```python
from build123d import *

# Parameters (mm, degrees)
BOSS_EXTRUDE1_DEPTH                           = 50.8
CSK_FOR_8_FLAT_HEAD_MACHINE_SCREW1_AT_2_COUNT = 2
CSK_FOR_8_FLAT_HEAD_MACHINE_SCREW1_AT_2_PITCH = 31.75


with BuildPart() as part:
    # Sketch1 → Boss-Extrude1 (new body)
    with BuildSketch(Plane.XY):
        Polygon((0, 0), (0, 38.1), (3.175, 38.1), (3.175, 3.175), (92.075, 3.175), (92.075, 25.4), (95.25, 25.4), (95.25, 0), align=None)
    extrude(amount=BOSS_EXTRUDE1_DEPTH)

    # Sketch3 → CSK for #8 Flat Head Machine Screw1 (revolve, cut)
    with BuildSketch(Plane(origin=(3.175, 31.75, 41.275), x_dir=(0, 0, -1), z_dir=(0, 1, 0))):
        Polygon((0, 0), (0, 3.175), (2.2479, 3.175), (2.2479, 2.26450021), (4.2164, 0), align=None)
    csk_for_8_flat_head_machine_screw1 = revolve(axis=Axis((9.525, 31.75, 41.275), (-1, 0, 0)), mode=Mode.SUBTRACT)

    # CSK for #8 Flat Head Machine Screw1 at 2: CSK for #8 Flat Head Machine Screw1 ×2
    with Locations(*[(0, 0, -i * CSK_FOR_8_FLAT_HEAD_MACHINE_SCREW1_AT_2_PITCH) for i in range(1, CSK_FOR_8_FLAT_HEAD_MACHINE_SCREW1_AT_2_COUNT)]):
        add(csk_for_8_flat_head_machine_screw1, mode=Mode.SUBTRACT)


solid = part.part
```
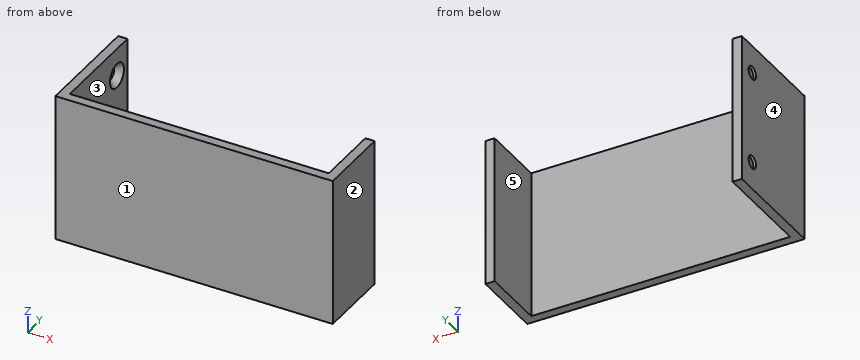
Source: CAD feature listing. Evaluate the final solid. Frame: model axes, mm. Face numbers are marked on the shaded views. A direction names the side the tool comes from. Give positions to 0.01 mm unless a question says otherwise; leave off trailing zeros. Loops run counter-clockwise (first coordinate to the right, second up) from the corner with the lowest first, then second, coordinate; pieces in that order, holes last. Notation, with made-up numbers: (19.5, -12.5) - (56.5, -12.5) arc R17 ccw to (56.5, 17.5) - close; hole circle Ø2 at (24.5, 21). An arc over 180 degrees is marked (long way). Use CSV: the item, a comma, the result in double quotes. Start each with the question number.
1. Section A-A (y = 31.75). Output: boundary loops of the cut face in (x, z) (1 decimal), then the cut area to 3 significant figures.
2. Section B-B (z = 35.5). Output: boundary loops of the cut face in (x, y) (3 decimals), then the cut area to 3 significant figures.
3. Draft query along X for the marked faces 1, 2 and 3. Return one class per face: +X half, -X half, draft (parallel to the pull), parting line (faces both ways), or undercut.
4. Ray query, L1, parallel to Z at x = 0.5, y = 31.75; L2, parallel to X at y = 11, z = 12.5 (3 decimals); L3, parallel to X at y = 35.5, z = 5 (3 decimals). Return the intervals inside material, ascending.
5. Section C-C (y = 4.5). Output: boundary loops of the cut face in (x, z) (3 decimals).
6. Reachability of the marked faces 4 and 5 from +Z, -Z, +X, -X, +Y, -Y: full face, straight path, thin tool, end or side. Return the list, or none.
7. Pin query (flat end, axial travel): pin 1 (2.5 mm diameter, centred on x = 94, z = 29, fed in from +Y); pin 2 (5 mm diameter, centred on x = 57.5, z = 16.5, fed in from +Y) (3 decimals). Return the tip coordinate at first contact, or that it passes through.
8. Section D-D (x = 40.5). Output: boundary loops of the cut face in (y, z) (3 decimals), then the cut area to 3 significant figures.
Response:
1,outline,"(0, 0) - (3.2, 0) - (3.2, 5.3) - (0.9, 7.3) - (0, 7.3) - close; (0, 11.8) - (0.9, 11.8) - (3.2, 13.7) - (3.2, 37.1) - (0.9, 39) - (0, 39) - close; (0, 43.5) - (0.9, 43.5) - (3.2, 45.5) - (3.2, 50.8) - (0, 50.8) - close"
1,area,"124 mm²"
2,outline,"(0, 0) - (95.25, 0) - (95.25, 25.4) - (92.075, 25.4) - (92.075, 3.175) - (3.175, 3.175) - (3.175, 38.1) - (0, 38.1) - close"
2,area,"484 mm²"
3,face 1,"draft"
3,face 2,"+X half"
3,face 3,"undercut"
4,L1,"0 to 7.28, 11.77 to 39.03, 43.52 to 50.8"
4,L2,"0 to 3.175, 92.075 to 95.25"
4,L3,"0 to 3.175"
5,outline,"(0, 0) - (3.175, 0) - (3.175, 50.8) - (0, 50.8) - close; (92.075, 0) - (95.25, 0) - (95.25, 50.8) - (92.075, 50.8) - close"
6,face 4,"+Z, -Z, -X, +Y, -Y"
6,face 5,"+Z, -Z, +Y"
7,pin 1,"y = 25.4"
7,pin 2,"y = 3.175"
8,outline,"(0, 0) - (3.175, 0) - (3.175, 50.8) - (0, 50.8) - close"
8,area,"161 mm²"
